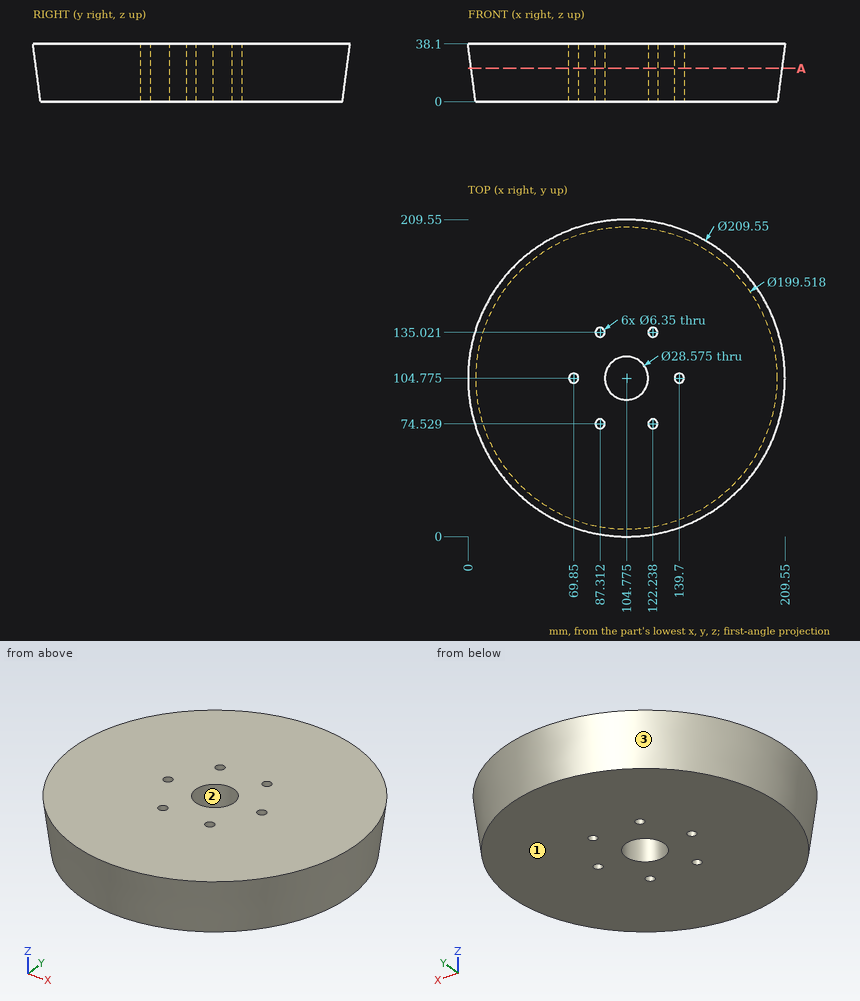
Verification items for this drawing (mm, ordinates from the low corner). Coordinates: 2 decimals unless noted, no trailing zeros.
Item 1: Sectioned sample at A-A, the plane z = 22. Count the separate pieces of the cut face and the enclosed holes in it, then the cut area to 3 significant figures.
Item 2: Thickness scan on line 1 (Y direction, x = 87.5, z = 11); line 2 (X direction, y = 103, z = 21.5); line 3 (Y direction, x = 87, z = 16). Record the ranges inside material, lowest first.
Item 3: Go/stop test with flat-tipped pins: pin 1 Ø4 at (x, z) = (160, 10) entering from +Y; pin 2 Ø3 at (x, z) = (60.5, 27) entering from +Y; pin 3 Ø12 at (x, z) = (34, 14) entering from -Y (1 decimal). Record where each tip stops, or that it passes through.
Item 4: Release check for a two-part mould opening along X. For the marked faces 1, 2 and 3 record: released by +X, released by -X, zero draft, split by the parting line, or undercut.
Check result:
1. separate pieces: 1
1. enclosed holes: 7
1. area: 32,300 mm2
2. line 1: y = 5.05 to 71.36, 77.7 to 131.85, 138.19 to 204.5
2. line 2: x = 2.2 to 67.22, 72.48 to 90.6, 118.95 to 137.07, 142.33 to 207.35
2. line 3: y = 4.47 to 71.37, 77.69 to 131.86, 138.18 to 205.08
3. pin 1: stops at y = 190.74
3. pin 2: stops at y = 198.85
3. pin 3: stops at y = 26.4
4. face 1: zero draft
4. face 2: undercut
4. face 3: split by the parting line
